Part model, mm, in its own coordinate system. Round coordinates to 2 decimals unless told otherwise and drop trailing zeros. Write each loop counter-clockwise with the first axis right and the second up, starting at its lowest first coordinate (ties: lowest second). Pieces come first, ordered by that corner, then holes. Notation, with made-up numbers: (83.5, 60.5) -> (117.5, 60.5) arc R26 cw to (117.5, 77.5) -> close; hole circle Ø2 at (-27.5, 39). An arc over 180 degrees is marked (long way). Return JSON: item names as keys, results as strings. Group by question number.
(1) Saw through at C-C (x = 12). List the corners of the cut face in (y, z), plus the area to 3 significant figures.
(2) Saw through at A-A (z = 0.7). List the corners of the cut face in (x, y).
(3) Saw through at B-B (y = 79.5). List the corners of the cut face in (x, z).
(4) Drop flat-ended pins along their axis: pin 1 Ø4 at (x, y) = (71.5, 44) entering from -Z; pin 2 Ø1.2 at (x, z) = (1, 1) entering from +Y; pin 3 Ø1 at (y, z) = (72.5, 1) entering from -X; pin 4 Ø1.2 at (x, z) = (4.5, 1.5) entering from -Y. Give the stop position or say it passes through.
(5) Drill centre lines: L1, parallel to Y at x = 77, z = 1.6; L2, parallel to Y at x = 17, z = 2.45. Where is each one in solid material? Low to high. Write a range as from..to.
Autodesk Fusion 360 part; units mm, degrees
sketch "Sketch1" plane through (0, 0, 0) normal (0, 0, 1) x (1, 0, 0)
  line L0 (-10, 20) -> (-10, 60)
  line L1 (90, 60) -> (90, 20)
  line L2 (90, 20) -> (-10, 60) construction
  line L3 (-10, 20) -> (90, 60) construction
  line L4 (60, -10) -> (20, -10)
  line L5 (20, 90) -> (60, 90)
  line L6 (60, -10) -> (20, 90) construction
  line L7 (20, -10) -> (60, 90) construction
  line L8 (-10, 60) -> (10, 60)
  line L9 (70, 60) -> (90, 60)
  line L10 (60, 90) -> (60, 70)
  line L11 (60, 10) -> (60, -10)
  line L12 (90, 20) -> (70, 20)
  line L13 (10, 20) -> (-10, 20)
  line L14 (20, -10) -> (20, 10)
  line L15 (20, 70) -> (20, 90)
  arc A0 (10, 60) -> (20, 70) centre (10, 70) ccw
  arc A1 (60, 70) -> (70, 60) centre (70, 70) ccw
  arc A2 (70, 20) -> (60, 10) centre (70, 10) ccw
  arc A3 (20, 10) -> (10, 20) centre (10, 10) ccw
  point P0 (40, 40)
  point P1 (40, 40)
  dimension "d1" = 100
  dimension "d2" = 40
  dimension "d3" = 40
  dimension "d4" = 100
  dimension "d5" = 10
  dimension "d6" = 10
  dimension "d7" = 10
  dimension "d8" = 10
extrude "Extrude1" add sketch "Sketch1" along normal blind 2.5
fillet "Fillet1" radius 5 1 edges at (60, -10, 1.25)
fillet "Fillet2" radius 5 1 edges at (20, -10, 1.25)
fillet "Fillet3" radius 5 1 edges at (-10, 20, 1.25)
fillet "Fillet4" radius 5 2 edges at (-10, 60, 1.25) (20, 90, 1.25)
fillet "Fillet5" radius 5 2 edges at (60, 90, 1.25) (90, 60, 1.25)
fillet "Fillet6" radius 5 1 edges at (90, 20, 1.25)
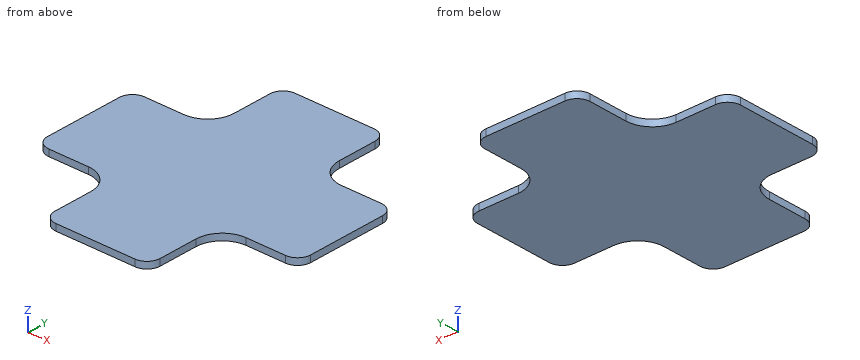
Computed values:
{
 "1": {"outline": "(19.8, 0) -> (60.2, 0) -> (60.2, 2.5) -> (19.8, 2.5) -> close", "area": "101 mm2"},
 "2": {"outline": "(-10, 25) arc R5 ccw to (-5, 20) -> (10, 20) arc R10 cw to (20, 10) -> (20, -5) arc R5 ccw to (25, -10) -> (55, -10) arc R5 ccw to (60, -5) -> (60, 10) arc R10 cw to (70, 20) -> (85, 20) arc R5 ccw to (90, 25) -> (90, 55) arc R5 ccw to (85, 60) -> (70, 60) arc R10 cw to (60, 70) -> (60, 85) arc R5 ccw to (55, 90) -> (25, 90) arc R5 ccw to (20, 85) -> (20, 70) arc R10 cw to (10, 60) -> (-5, 60) arc R5 ccw to (-10, 55) -> close"},
 "3": {"outline": "(20, 0) -> (60, 0) -> (60, 2.5) -> (20, 2.5) -> close"},
 "4": {"pin 1": "z = 0", "pin 2": "y = 60", "pin 3": "x = 20", "pin 4": "y = 20"},
 "5": {"L1": "20..60", "L2": "17.14..62.86"}
}
